```python
from build123d import *

# Parameters (mm, degrees)
SKETCH_1_R      = 2
SKETCH_1_R_2    = 1
EXTRUDE_1_DEPTH = 3
FILLET_1_R      = 1


with BuildPart() as part:
    # 草图1 → 凸台-拉伸1 (new body)
    with BuildSketch(Plane.XY):
        with BuildLine():
            Line((66.731946056, 69.612461713), (73.815819619, 62.821713952))
            Line((73.815819619, 62.821713952), (3.432687046, -3.63547241))
            ThreePointArc((3.432687046, -3.63547241), (-3.460067431, -3.609422859), (-3.777206949, 3.276081144))
            Line((-3.777206949, 3.276081144), (61.945586102, 79.052162289))
            ThreePointArc((61.945586102, 79.052162289), (74.586475775, 81.109748207), (78.884235331, 69.045129923))
            Line((78.884235331, 69.045129923), (72.268053944, 75.387538287))
            ThreePointArc((72.268053944, 75.387538287), (66.612461713, 75.268053944), (66.731946056, 69.612461713))
        make_face()
        Circle(SKETCH_1_R, mode=Mode.SUBTRACT)
        with Locations((30.891832327, 25)):
            Circle(SKETCH_1_R_2, mode=Mode.SUBTRACT)
    extrude(amount=EXTRUDE_1_DEPTH)

    # 圆角1
    fillet_1_edges = [part.edges().sort_by_distance(p)[0] for p in [
        (73.815819619, 62.821713952, 1.5),
        (78.884235331, 69.045129923, 1.5),
    ]]
    fillet(fillet_1_edges, radius=FILLET_1_R)


solid = part.part
```
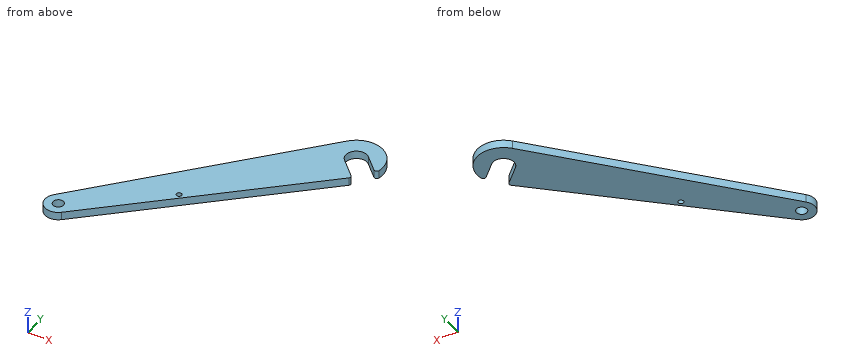
The listing builds one solid part. Answer for the finished solid, in the listing's coordinates (mm). Round coordinates to 2 decimals unless told otherwise and drop trailing zeros. Loops run counter-clockwise (first coordinate to the right, second up) from the corner with the lowest first, then second, coordinate; pieces in that order, holes last.
Q1. Section C-C, the plane y = 72.5 is taken. Determine the outline of the cut face in (x, z), then the cut area to 3 significant figures.
Q2. Section A-A, the plane x = 0.5 is taken. Determine the outline of the cut face in (y, z), then the cut area to 3 significant figures.
Q3. Given pin 1 Ø1 at (x, z) = (26.5, 2) entering from +Y; pin 2 Ø1 at (x, z) = (46, 1) entering from -Y, each flat-ended and moving along its own axis, determine where each tip first touches the part or whether it passes through.
Q4. Section D-D, the plane x = 19.5 is taken. Determine the outline of the cut face in (y, z).
Q5. Find the intervals of material crossed by line 1 (X direction, y = 71.5, z = 2); line 2 (X direction, y = 75.5, z = 0.35); line 3 (Y direction, x = 71, z = 2), in increasing order.
Q6. Section B-B, the plane z = 2.25 is taken. Determine the outline of the cut face in (x, y).
Completed:
1. outline: (56.26, 0) - (65.5, 0) - (65.5, 3) - (56.26, 3) - close; (75.28, 0) - (79.5, 0) - (79.5, 3) - (75.28, 3) - close
1. area: 40.4 mm2
2. outline: (-4.97, 0) - (-1.94, 0) - (-1.94, 3) - (-4.97, 3) - close; (1.94, 0) - (8.21, 0) - (8.21, 3) - (1.94, 3) - close
2. area: 27.9 mm2
3. pin 1: stops at y = 38.76
3. pin 2: stops at y = 36.09
4. outline: (11.54, 0) - (30.11, 0) - (30.11, 3) - (11.54, 3) - close
5. line 1: x = 55.4 to 65.63, 76.32 to 79.45
5. line 2: x = 58.86 to 66.85, 72.15 to 79.04
5. line 3: y = 60.16 to 65.52, 76.21 to 82.39
6. outline: (-3.78, 3.28) arc R5 ccw to (3.43, -3.64) - (73.05, 62.1) arc R1 ccw to (73.06, 63.55) - (66.73, 69.61) arc R4 cw to (72.27, 75.39) - (77.67, 70.21) arc R1 ccw to (79.35, 70.76) arc R10 ccw to (61.95, 79.05) - close; hole circle Ø4 at (0, 0); hole circle Ø2 at (30.89, 25)
